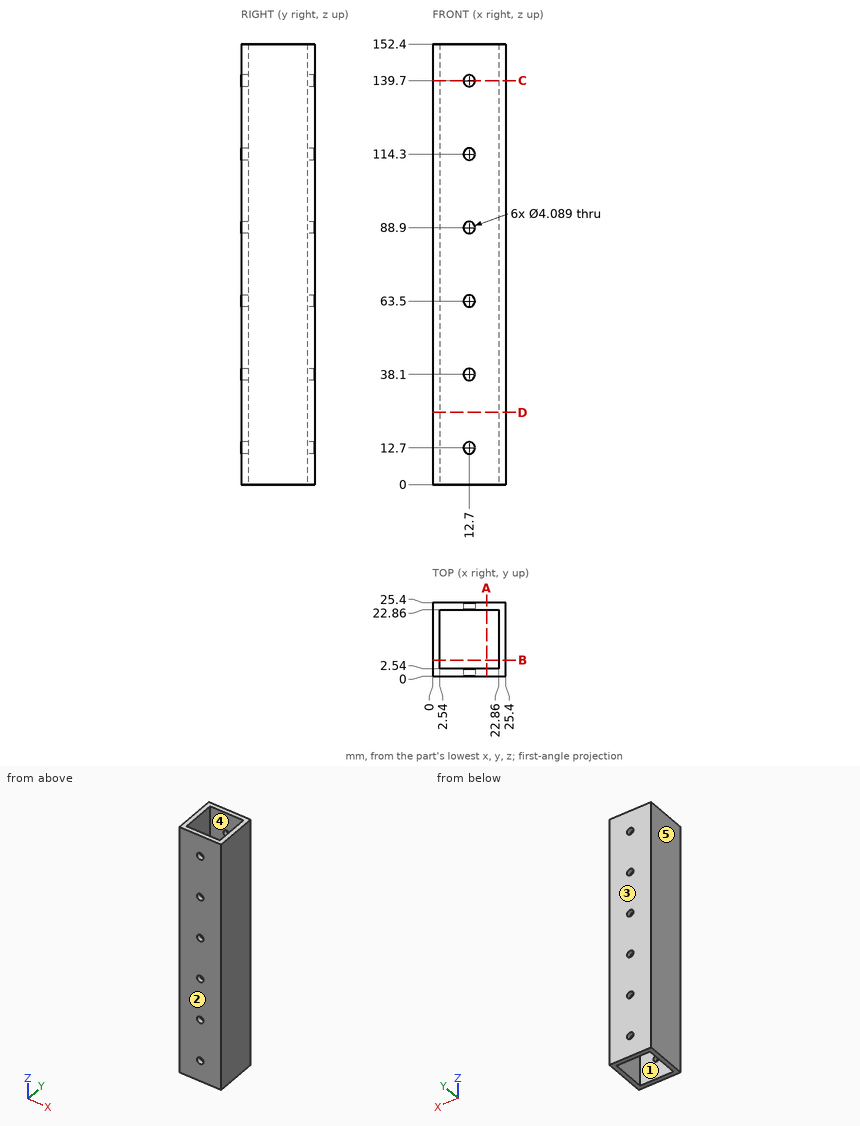
The drawing under review shows one solid part. Ordinate dimensions are in mm from its lowest x, y, z. A direction names the side the tool comes from. Coordinates: 2 decimals unless noted, no trailing zeros. Order: outer loops, then holes, each group sorted by start corner. A loop starts at its lowest first (then second) coordinate and runs counter-clockwise, first axis right, second up. Notation, with made-up numbers: (24, -21.75) -> (53, -21.75) arc R33 cw to (53, 7.25) -> close; hole circle Ø1 at (-18.5, 49). An arc over 180 degrees is marked (long way). Return JSON: item names as keys, results as strings.
1. Machinability: for the marked faces 1 and 2, which of the approach directions +Z, -Z, +X, -X, +Y, -Y give a long, thin tool a straight path to every point of the face, cutting with its end or side? Answer none if there is none.
Answer block:
{"face 1": "+Z, -Z", "face 2": "+Z, -Z, +X, -X, -Y"}
2. We need section A-A on x = 18.75. Write out the cut boundary in (y, z).
Answer block:
{"outline": "(0, 0) -> (2.54, 0) -> (2.54, 152.4) -> (0, 152.4) -> close; (22.86, 0) -> (25.4, 0) -> (25.4, 152.4) -> (22.86, 152.4) -> close"}
3. The part is to be moulded in two halves that separate along Y. For the marked faces 3, 4 and 5, say which applies: +Y half, -Y half, draft (parallel to the pull), parting line (faces both ways), or undercut.
Answer block:
{"face 3": "+Y half", "face 4": "undercut", "face 5": "draft"}
4. For line 1 (Y direction, x = 16.75, z = 118.5); line 2 (X direction, y = 23.5, z = 88.9) (1 decimal), list the stretches that pass through material, from the lowest coordinate up. Write a range as from..to.
Answer block:
{"line 1": "0..2.54, 22.86..25.4", "line 2": "0..10.7, 14.7..25.4"}
5. We need section C-C on z = 139.7. Write out the cut boundary in (x, y) (1 decimal).
Answer block:
{"outline": "(0, 0) -> (10.7, 0) -> (10.7, 2.5) -> (2.5, 2.5) -> (2.5, 22.9) -> (10.7, 22.9) -> (10.7, 25.4) -> (0, 25.4) -> close; (14.7, 0) -> (25.4, 0) -> (25.4, 25.4) -> (14.7, 25.4) -> (14.7, 22.9) -> (22.9, 22.9) -> (22.9, 2.5) -> (14.7, 2.5) -> close"}
6. We need section D-D on z = 25. Write out the cut boundary in (x, y), and give its area (3 significant figures).
Answer block:
{"outline": "(0, 0) -> (25.4, 0) -> (25.4, 25.4) -> (0, 25.4) -> close; hole (2.54, 2.54) -> (22.86, 2.54) -> (22.86, 22.86) -> (2.54, 22.86) -> close", "area": "232 mm²"}
